```python
from build123d import *

# Parameters (mm, degrees)
SKETCH1_W               = 25
SKETCH1_H               = 25
BOSS_EXTRUDE1_DEPTH     = 15
SKETCH2_R               = 11.21
SKETCH2_R_2             = 9.71
CUT_EXTRUDE1_DEPTH      = 4
CUT_EXTRUDE4_REACH      = 33.721
CUT_EXTRUDE4_END_RADIUS = 11.21
SKETCH4_R               = 8.5


with BuildPart() as part:
    # Sketch1 → Boss-Extrude1 (new body)
    with BuildSketch(Plane(origin=(0, 0, 0), x_dir=(0, 0, -1), z_dir=(1, 0, 0))):
        Rectangle(SKETCH1_W, SKETCH1_H)
    extrude(amount=BOSS_EXTRUDE1_DEPTH)

    # Sketch2 → Cut-Extrude1 (cut)
    with BuildSketch(Plane.ZY):
        Circle(SKETCH2_R)
        Circle(SKETCH2_R_2, mode=Mode.SUBTRACT)
    extrude(amount=-CUT_EXTRUDE1_DEPTH, mode=Mode.SUBTRACT)

    # Cut-Extrude4: up to this cylinder (the profile starts outside it)
    cut_extrude4_end = Plane(origin=(7.008609, 0, 0), z_dir=(-1, 0, 0)) * Cylinder(CUT_EXTRUDE4_END_RADIUS, 90.862, mode=Mode.PRIVATE)
    # Sketch4 → Cut-Extrude4 (cut, up to the surface)
    with BuildSketch(Plane.XY.offset(12.5), mode=Mode.PRIVATE) as cut_extrude4_sk1:
        with Locations((7.008609298, 0)):
            Circle(SKETCH4_R)
    cut_extrude4_tool1 = extrude(cut_extrude4_sk1.sketch, amount=-CUT_EXTRUDE4_REACH, mode=Mode.PRIVATE) - cut_extrude4_end
    add(cut_extrude4_tool1.solids().sort_by_distance((7.008609, 0, 12.5))[0], mode=Mode.SUBTRACT)


solid = part.part
```
Build history of the part. All positions in model axes, mm. A direction names the side the tool comes from. Give positions to 0.01 mm unless a question says otherwise; leave off trailing zeros. Loops run counter-clockwise (first coordinate to the right, second up) from the corner with the lowest first, then second, coordinate; pieces in that order, holes last. Notation, with made-up numbers: (25.5, 4.25) - (76.5, 4.25) arc R20 ccw to (76.5, 29.25) - close; hole circle Ø3 at (48, 56.5). An arc over 180 degrees is marked (long way). Use a Markdown table: item, result.
(1) Band-saw the part on A-A (y = 7.5). Give the cut face in (x, z), and give its area (3 significant figures).
Taken from the geometry:
| item | result |
|---|---|
| outline | (0, -12.5) - (15, -12.5) - (15, 12.5) - (11.01, 12.5) - (11.01, 8.33) - (4, 8.33) - (4, 6.17) - (0, 6.17) - (0, -6.17) - (4, -6.17) - (4, -8.33) - (0, -8.33) - close; (0, 8.33) - (3.01, 8.33) - (3.01, 12.5) - (0, 12.5) - close |
| area | 324 mm2 |
(2) Band-saw the part on B-B (y = 0). Give the cut face in (x, z).
Taken from the geometry:
| item | result |
|---|---|
| outline | (0, -12.5) - (15, -12.5) - (15, 11.21) - (4, 11.21) - (4, 9.71) - (0, 9.71) - (0, -9.71) - (4, -9.71) - (4, -11.21) - (0, -11.21) - close |
(3) Band-saw the part on C-C (z = 0). Give the cut face in (x, y), and give its area (3 significant figures).
Taken from the geometry:
| item | result |
|---|---|
| outline | (0, -12.5) - (15, -12.5) - (15, 12.5) - (0, 12.5) - (0, 11.21) - (4, 11.21) - (4, 9.71) - (0, 9.71) - (0, -9.71) - (4, -9.71) - (4, -11.21) - (0, -11.21) - close |
| area | 363 mm2 |
(4) Band-saw the part on D-D (x = 9). Give the cut face in (y, z).
Taken from the geometry:
| item | result |
|---|---|
| outline | (-12.5, -12.5) - (12.5, -12.5) - (12.5, 12.5) - (8.26, 12.5) - (8.26, 7.57) arc R11.21 ccw to (-8.26, 7.57) - (-8.26, 12.5) - (-12.5, 12.5) - close |
(5) Which spindle directions (+Z, -Z, +X, -X, +Y, -Y) get a long thin tool onto all of the face, cutting with end or side? Do faces 4 (the face through (0, 3, -11)), 5 (the face through (1.972, 0.423, -11.202)), 6 (the face through (7.954, -8.447, 10.517)). Say none if no direction does.
Taken from the geometry:
| item | result |
|---|---|
| face 4 | +Z, -Z, -X, +Y, -Y |
| face 5 | -X |
| face 6 | +Z |
(6) Drop flat-ended pins along their axis: pin 1 Ø8 at (y, z) = (-6, -6.5) entering from -X; pin 2 Ø1.5 at (x, y) = (6, 7) entering from +Z; pin 3 Ø5 at (x, y) = (7.5, -5) entering from +Z. Give the stop position or say it passes through.
Taken from the geometry:
| item | result |
|---|---|
| pin 1 | x = 0 |
| pin 2 | z = 9.31 |
| pin 3 | z = 10.93 |
(7) Wall check: line 1 along Y through (x, z) = (2.1, 0); line 2 along Y through (x, z) = (1.25, -1.25); line 3 along X through (y, z) = (-10.5, -2.25). Give the ranges that are in metal, low to high.
Taken from the geometry:
| item | result |
|---|---|
| line 1 | -12.5 to -11.21, -9.71 to 9.71, 11.21 to 12.5 |
| line 2 | -12.5 to -11.14, -9.63 to 9.63, 11.14 to 12.5 |
| line 3 | 4 to 15 |
(8) Pull direction Z, two halves, no side cores. Call faces 1 (the face through (7, -12.5, 0)), 2 (the face through (4, 10, 0)), 3 (the face through (7, -10, 12.5)): +Z half, -Z half, draft (parallel to the pull), parting line (faces both ways), or undercut.
Taken from the geometry:
| item | result |
|---|---|
| face 1 | draft |
| face 2 | undercut |
| face 3 | +Z half |
